Part model, mm, in its own coordinate system. A direction names the side the tool comes from. Give positions to 0.01 mm unless a question says otherwise; leave off trailing zeros. Write each loop counter-clockwise with the first axis right and the second up, starting at its lowest first coordinate (ties: lowest second). Pieces come first, ordered by that corner, then holes. Notation, with made-up numbers: (-29, 64.25) - (-3, 64.25) arc R20 ccw to (-3, 79.25) - close; hole circle Ø1 at (80, -37.75). An arc over 180 degrees is marked (long way). Answer in a Markdown table with one row per item. Add a question column.
1. Probe line 1 along X through (y, z) = (-5.75, 0.75); line 2 along Y through (x, z) = (5, -3.5); line 3 along Z through (x, y) = (3.75, 5.5). List the from-to ranges inside material, lowest first.
2. Band-saw the part on C-C on z = 2.75. Write the cut outline in (x, y).
3. Drop flat-ended pins along their axis: pin 1 Ø1.5 at (x, y) = (-4, -1) entering from +Z; pin 2 Ø6 at (x, z) = (-4.5, -3) entering from +Y; pin 3 Ø6 at (x, y) = (1, 5) entering from -Z; pin 4 Ø1.5 at (x, z) = (0.5, -1) entering from -Y. Give the stop position or say it passes through.
4. Band-saw the part on A-A on y = 0. Write the cut outline in (x, z), plus the area to 3 significant figures.
5. Band-saw the part on B-B on x = 2.75. Write the cut outline in (y, z).
6. Which spindle directions (+Z, -Z, +X, -X, +Y, -Y) get a long thin tool onto all of the face, cutting with end or side? Do faces 1 (the cylindrical face through (-4, 2, 0)), 2 (the flat face through (2.96, -6.72, 3.95)). Say none if no direction does.
7. Band-saw the part on D-D on y = 2.75. Write the cut outline in (x, z).
```python
from build123d import *

# Parameters (mm, degrees)
BOSS_EXTRUDE1_DEPTH = 6
SKETCH2_R           = 2
BOSS_EXTRUDE2_DEPTH = 8


with BuildPart() as part:
    # Sketch1 → Boss-Extrude1 (new body)
    with BuildSketch(Plane(origin=(0, 0, 0), x_dir=(0, 0, -1), z_dir=(1, 0, 0))):
        Polygon((0, -9), (7.794228634, -4.5), (7.794228634, 4.5), (0, 9), (-7.794228634, 4.5), (-7.794228634, -4.5), align=None)
    extrude(amount=BOSS_EXTRUDE1_DEPTH)

    # Sketch2 → Boss-Extrude2 (add)
    with BuildSketch(Plane.ZY):
        with Locations(Location((0, 0, 0), (0, 0, 180))):
            Circle(SKETCH2_R)
    extrude(amount=BOSS_EXTRUDE2_DEPTH)


solid = part.part
```
Values:
| question | item | result |
|---|---|---|
| 1 | line 1 | x = 0 to 6 |
| 1 | line 2 | y = -6.98 to 6.98 |
| 1 | line 3 | z = -6.06 to 6.06 |
| 2 | outline | (0, -7.41) - (6, -7.41) - (6, 7.41) - (0, 7.41) - close |
| 3 | pin 1 | stops at z = 1.98 |
| 3 | pin 2 | stops at y = 2 |
| 3 | pin 3 | stops at z = -7.79 |
| 3 | pin 4 | stops at y = -8.86 |
| 4 | outline | (-8, -2) - (0, -2) - (0, -7.79) - (6, -7.79) - (6, 7.79) - (0, 7.79) - (0, 2) - (-8, 2) - close |
| 4 | area | 126 mm² |
| 5 | outline | (-9, 0) - (-4.5, -7.79) - (4.5, -7.79) - (9, 0) - (4.5, 7.79) - (-4.5, 7.79) - close |
| 6 | face 1 | -X |
| 6 | face 2 | +Z, +X, -X, -Y |
| 7 | outline | (0, -7.79) - (6, -7.79) - (6, 7.79) - (0, 7.79) - close |
